Could you check a few things on this model? Use its own coordinates, in mm. Face numbers are marked on the shaded views. A direction names the side the tool comes from. Round coordinates to 2 decimals unless told otherwise and drop trailing zeros. Write each loop counter-clockwise with the first axis right and the second up, starting at its lowest first coordinate (ties: lowest second). Pieces come first, ordered by that corner, then holes. Notation, with made-up numbers: M -22,65.5 L -14,65.5 A17 cw -14,79.5 Z; hole C 39,-6.75 d7. An arc over 180 degrees is marked long. One line per question, with ' | ' between items. Start each with the question number.
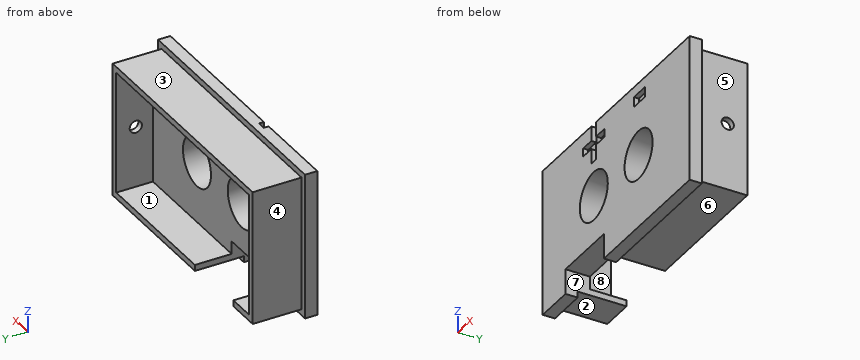
```python
from build123d import *

# Parameters (mm, degrees)
SKETCH1_W           = 42
SKETCH1_H           = 24
BOSS_EXTRUDE1_DEPTH = 2
BOSS_EXTRUDE2_DEPTH = 8
CUT_EXTRUDE1_DEPTH  = 6
CUT_EXTRUDE2_REACH  = 51.396
SKETCH2_R           = 4
SKETCH3_W           = 3.111111111
SKETCH3_H           = 1.652777778
CUT_EXTRUDE3_DEPTH  = 0.8
CUT_EXTRUDE4_REACH  = 51.396
SKETCH4_W           = 11
SKETCH4_H           = 4.114457091
CUT_EXTRUDE5_REACH  = 50.549
SKETCH5_R           = 1


with BuildPart() as part:
    # Sketch1 → Boss-Extrude1 (new body)
    with BuildSketch(Plane(origin=(0, 0, 0), x_dir=(1, 0, 0), z_dir=(0, 1, 0))):
        with Locations((21, 12)):
            Rectangle(SKETCH1_W, SKETCH1_H)
    extrude(amount=BOSS_EXTRUDE1_DEPTH)

    # 3DSketch1 → Boss-Extrude2 (add)
    with BuildSketch(Plane(origin=(1, 2, -1), x_dir=(0.876215908676647, 0, -0.4819187497721558), z_dir=(0, -1, 0))):
        Polygon((0, 0), (35.048636347, 19.276749991), (45.650848842, 0), (10.602212495, -19.276749991), align=None)
    extrude(amount=-BOSS_EXTRUDE2_DEPTH)

    # 3DSketch2 → Cut-Extrude1 (cut)
    with BuildSketch(Plane(origin=(2, 10, -2), x_dir=(0.8849182223819825, 0, -0.4657464328326223), z_dir=(0, -1, 0))):
        Polygon((0, 0), (33.626892451, 17.698364448), (42.941821107, 0), (9.314928657, -17.698364448), align=None)
    extrude(amount=CUT_EXTRUDE1_DEPTH, mode=Mode.SUBTRACT)

    # Sketch2 → Cut-Extrude2 (cut, up to next)
    with BuildSketch(Plane.XZ, mode=Mode.PRIVATE) as cut_extrude2_sk1:
        with Locations(Location((27.4, -12, 0), (0, 0, 270))):
            Circle(SKETCH2_R)
    cut_extrude2_tool1 = extrude(cut_extrude2_sk1.sketch, amount=-CUT_EXTRUDE2_REACH, mode=Mode.PRIVATE) & part.part
    # Sketch2 → Cut-Extrude2 (cut, up to next)
    with BuildSketch(Plane.XZ, mode=Mode.PRIVATE) as cut_extrude2_sk2:
        with Locations(Location((14.6, -12, 0), (0, 0, 270))):
            Circle(SKETCH2_R)
    cut_extrude2_tool2 = extrude(cut_extrude2_sk2.sketch, amount=-CUT_EXTRUDE2_REACH, mode=Mode.PRIVATE) & part.part
    add(cut_extrude2_tool1.solids().sort_by_distance((27.4, 0, -12))[0], mode=Mode.SUBTRACT)
    add(cut_extrude2_tool2.solids().sort_by_distance((14.6, 0, -12))[0], mode=Mode.SUBTRACT)

    # Sketch3 → Cut-Extrude3 (cut)
    with BuildSketch(Plane.XZ):
        Polygon((13.902777778, -6.222222222), (15.263888889, -6.222222222), (15.263888889, -3.791666667), (17.597222222, -3.791666667), (17.597222222, -2.430555556), (15.263888889, -2.430555556), (15.263888889, 0), (13.902777778, 0), (13.902777778, -2.430555556), (11.569444444, -2.430555556), (11.569444444, -3.791666667), (13.902777778, -3.791666667), align=None)
        with Locations((27.611111112, -2.479166667)):
            Rectangle(SKETCH3_W, SKETCH3_H)
    extrude(amount=-CUT_EXTRUDE3_DEPTH, mode=Mode.SUBTRACT)

    # Sketch4 → Cut-Extrude4 (cut, up to next)
    with BuildSketch(Plane.XZ, mode=Mode.PRIVATE) as cut_extrude4_sk1:
        with Locations((12, -21.942771455)):
            Rectangle(SKETCH4_W, SKETCH4_H)
    cut_extrude4_tool1 = extrude(cut_extrude4_sk1.sketch, amount=-CUT_EXTRUDE4_REACH, mode=Mode.PRIVATE) & part.part
    add(cut_extrude4_tool1.solids().sort_by_distance((12, 0, -21.942771))[0], mode=Mode.SUBTRACT)

    # Sketch5 → Cut-Extrude5 (cut, up to next)
    with BuildSketch(Plane(origin=(41, 0, 0), x_dir=(0, 0, -1), z_dir=(1, 0, 0)), mode=Mode.PRIVATE) as cut_extrude5_sk1:
        with Locations((12, 6.8)):
            Circle(SKETCH5_R)
    cut_extrude5_tool1 = extrude(cut_extrude5_sk1.sketch, amount=-CUT_EXTRUDE5_REACH, mode=Mode.PRIVATE) & part.part
    add(cut_extrude5_tool1.solids().sort_by_distance((41, 6.8, -12))[0], mode=Mode.SUBTRACT)


solid = part.part
```
1. Which directions (+Z, -Z, +X, -X, +Y, -Y) give clear straight access to the entire face, cutting with the end or side of a thin tool? Please do the marked faces 4, 5, 6, 7 and 8.
2. Suppose I cut it at D-D (x = 27.4). Write out the boundary of the cut face in (y, z), and give its area (3 significant figures).
3. I'm going to push flat-ended pins straight in: P1, Ø6, axis at y = 6.5, z = -14.5, coming from the +X side; P2, Ø0.9, axis at x = 16, y = 0.5, coming from the +Z side; P3, Ø2, axis at x = 33.5, y = 4, coming from the +Z side; P4, Ø2, axis at x = 34, z = -14.5, coming from the +Y side. Where does each tip first touch, or does it pass through?
4. Suppose I cut it at B-B (y = 2.75). Write out the boundary of the cut face in (x, z).
5. If we mould it in two halves opening along Z, with no side actions, what happens to the marked faces 1, 2 and 3? For each: released by +Z, released by -Z, zero draft, split by the parting line, or undercut.
6. I need wall thicknesses on line 1 along X through (y, z) = (1.1, -12); line 2 along X through (y, z) = (2.7, -12); line 3 along X through (y, z) = (8.25, -15.25). Which ranges of each line are inside material? Lowest first, please. Write a range as from..to.
7. Suppose I cut it at A-A (z = -12). Write out the boundary of the cut face in (x, y).
8. Suppose I cut it at C-C (z = -21.5). Write out the boundary of the cut face in (x, y), and give its area (3 significant figures).
Computed:
1) face 4: +Z, -Z, -X, +Y | face 5: +Z, -Z, +X, +Y | face 6: -Z, +X, -X, +Y | face 7: -Z, +Y, -Y | face 8: +Y
2) outline: M 0,-24 L 2,-24 L 2,-23 L 10,-23 L 10,-22 L 4,-22 L 4,-16 L 0,-16 Z; M 0,-8 L 4,-8 L 4,-2 L 10,-2 L 10,-1 L 2,-1 L 2,0 L 0,0 L 0,-1.65 L 0.8,-1.65 L 0.8,-3.31 L 0,-3.31 Z | area: 70.7 mm²
3) P1: stops at x = 41 | P2: stops at z = 0 | P3: stops at z = -1 | P4: stops at y = 4
4) outline: M 1,-23 L 6.5,-23 L 6.5,-19.89 L 17.5,-19.89 L 17.5,-23 L 41,-23 L 41,-1 L 1,-1 Z; hole C 14.6,-12 d8; hole C 27.4,-12 d8
5) face 1: undercut | face 2: released by -Z | face 3: released by +Z
6) line 1: x = 0..10.6, 18.6..23.4, 31.4..42 | line 2: x = 1..10.6, 18.6..23.4, 31.4..41 | line 3: x = 1..2, 40..41
7) outline: M 0,0 L 10.6,0 L 10.6,4 L 2,4 L 2,10 L 1,10 L 1,2 L 0,2 Z; M 18.6,0 L 23.4,0 L 23.4,4 L 18.6,4 Z; M 31.4,0 L 42,0 L 42,2 L 41,2 L 41,5.8 L 40,5.8 L 40,4 L 31.4,4 Z; M 40,7.8 L 41,7.8 L 41,10 L 40,10 Z
8) outline: M 0,0 L 6.5,0 L 6.5,4 L 2,4 L 2,10 L 1,10 L 1,2 L 0,2 Z; M 17.5,0 L 42,0 L 42,2 L 41,2 L 41,10 L 40,10 L 40,4 L 17.5,4 Z | area: 132 mm²
